Geometry check sheet. Reference: drawing and pictorial views, mm from the part's lowest x, y, z. A direction names the side the tool comes from. Give positions to 0.01 mm unless a question says otherwise; leave off trailing zeros. Write each loop counter-clockwise with the first axis right and the second up, starting at its lowest first coordinate (ties: lowest second). Pieces come first, ordered by that corner, then holes. Notation, with made-up numbers: (62, -35) -> (68, -35) arc R28 ccw to (68, -17) -> close; hole circle Ø1 at (74, 17). An arc over 180 degrees is marked (long way). Use a Markdown table: item, result. Add a question column.
1. Gauge pin test, flat ends, axial feed: P1, Ø1.2, axis at x = 7.5, y = 1.5, coming from the +Z side; P2, Ø1.2, axis at y = 0.5, z = 16.5, coming from the -X side (1 decimal); P3, Ø0.8, axis at y = 1.5, z = 13, coming from the +X side. Record the tip position at first contact, or that the pin passes through.
2. Cross-section at B-B (y = 2.2). Enter the section's corners in (x, z) (1 decimal).
3. Scan lines: probe 1 along X at (y, z) = (2.3, 16) (1 decimal); probe 2 along X at (y, z) = (0.95, 12) (1 decimal); probe 3 along Z at (x, y) = (11.75, 1.35). Record each from-to range of solid material in increasing order. Write a range as [from, to].
4. Cross-section at C-C (z = 8.25). Enter the section's corners in (x, y).
5. Set-up check for the marked faces 5, 6 and 7: record each of +Z, -Z, +X, -X, +Y, -Y from which the full face is reachable in a straight line by a thin tool's end or side.
6. Cross-section at A-A (z = 16). Enter the section's corners in (x, y) (1 decimal).
7. Release check for a two-part mould opening along X. For the marked faces 1, 2, 3 and 4 record: released by +X, released by -X, zero draft, split by the parting line, or undercut.
8. Cross-section at D-D (x = 16). Enter the section's corners in (y, z), then the cut area to 3 significant figures.
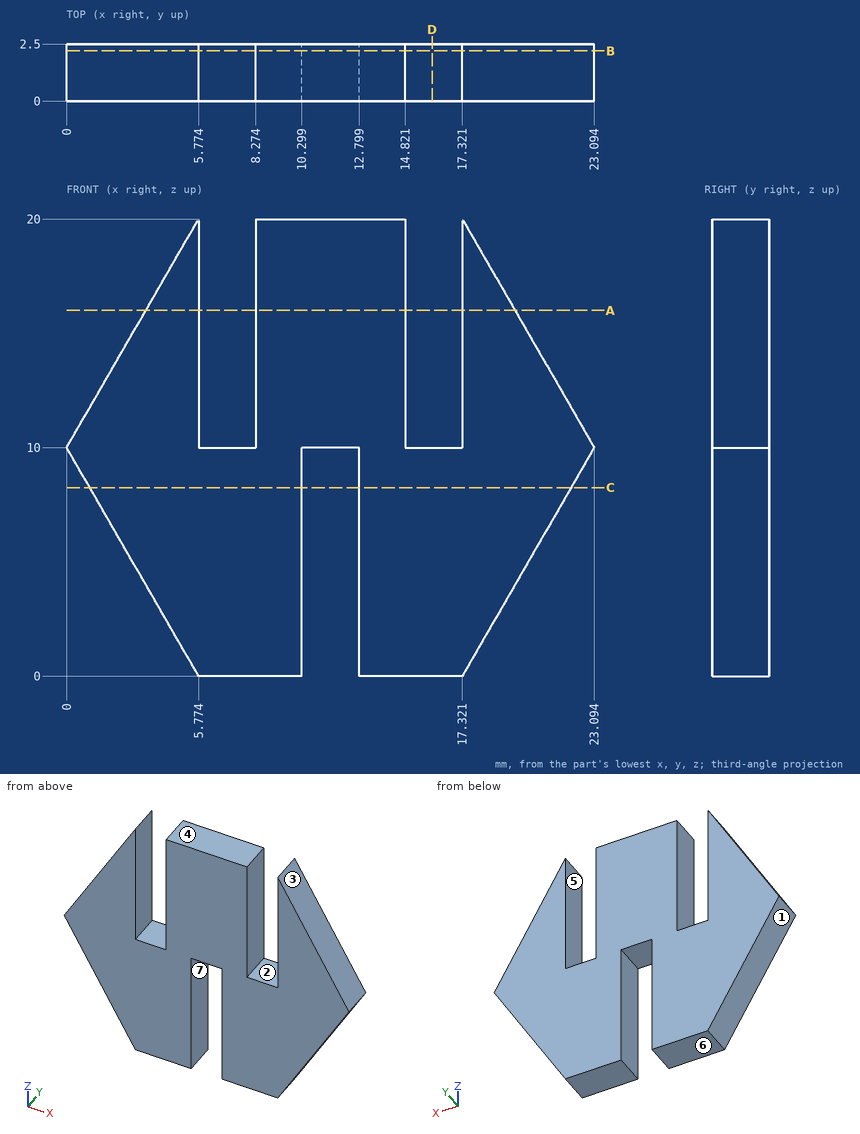
Worked answers:
| question | item | result |
|---|---|---|
| 1 | P1 | stops at z = 10 |
| 1 | P2 | stops at x = 3.4 |
| 1 | P3 | stops at x = 21.59 |
| 2 | outline | (0, 10) -> (5.8, 0) -> (10.3, 0) -> (10.3, 10) -> (12.8, 10) -> (12.8, 0) -> (17.3, 0) -> (23.1, 10) -> (17.3, 20) -> (17.3, 10) -> (14.8, 10) -> (14.8, 20) -> (8.3, 20) -> (8.3, 10) -> (5.8, 10) -> (5.8, 20) -> close |
| 3 | probe 1 | x = [3.5, 5.8], [8.3, 14.8], [17.3, 19.6] |
| 3 | probe 2 | x = [1.2, 5.8], [8.3, 14.8], [17.3, 21.9] |
| 3 | probe 3 | z = [10, 20] |
| 4 | outline | (1.01, 0) -> (10.3, 0) -> (10.3, 2.5) -> (1.01, 2.5) -> close; (12.8, 0) -> (22.08, 0) -> (22.08, 2.5) -> (12.8, 2.5) -> close |
| 5 | face 5 | +Z, +Y, -Y |
| 5 | face 6 | -Z, +X, -X, +Y, -Y |
| 5 | face 7 | -Z, +Y, -Y |
| 6 | outline | (3.5, 0) -> (5.8, 0) -> (5.8, 2.5) -> (3.5, 2.5) -> close; (8.3, 0) -> (14.8, 0) -> (14.8, 2.5) -> (8.3, 2.5) -> close; (17.3, 0) -> (19.6, 0) -> (19.6, 2.5) -> (17.3, 2.5) -> close |
| 7 | face 1 | released by -X |
| 7 | face 2 | undercut |
| 7 | face 3 | released by +X |
| 7 | face 4 | zero draft |
| 8 | outline | (0, 0) -> (2.5, 0) -> (2.5, 10) -> (0, 10) -> close |
| 8 | area | 25.0 mm² |
